```python
from build123d import *

# Parameters (mm, degrees)
SKETCH2_R           = 3
BOSS_EXTRUDE1_DEPTH = 4.7625
FILLET1_R           = 3.18


with BuildPart() as part:
    # Sketch2 → Boss-Extrude1 (new body)
    with BuildSketch(Plane.XY):
        Polygon((-31.10816412, 42.602538855), (8.89183588, 124.502538855), (48.89183588, 124.502538855), (88.89183588, 44.502538855), (88.89183588, 4.502538855), (-31.10816412, 4.502538855), align=None)
        with Locations(Location((28.89183588, 104.502538855, 0), (0, 0, 180))):
            Circle(SKETCH2_R, mode=Mode.SUBTRACT)
        with Locations(Location((28.89183588, 64.502538855, 0), (0, 0, 180))):
            Circle(SKETCH2_R, mode=Mode.SUBTRACT)
        with Locations(Location((-11.10816412, 23.552538855, 0), (0, 0, 180))):
            Circle(SKETCH2_R, mode=Mode.SUBTRACT)
        with Locations(Location((68.89183588, 23.552538855, 0), (0, 0, 180))):
            Circle(SKETCH2_R, mode=Mode.SUBTRACT)
        with Locations(Location((28.89183588, 23.552538855, 0), (0, 0, 180))):
            Circle(SKETCH2_R, mode=Mode.SUBTRACT)
    extrude(amount=BOSS_EXTRUDE1_DEPTH)

    # Fillet1
    fillet1_edges = [part.edges().sort_by_distance(p)[0] for p in [
        (-31.10816412, 42.602538855, 2.38125),
        (8.89183588, 124.502538855, 2.38125),
        (48.89183588, 124.502538855, 2.38125),
        (88.89183588, 44.502538855, 2.38125),
        (88.89183588, 4.502538855, 2.38125),
        (-31.10816412, 4.502538855, 2.38125),
    ]]
    fillet(fillet1_edges, radius=FILLET1_R)


solid = part.part
```
The model under review builds one solid part; all positions refer to its coordinate system, in mm. Give positions to 0.01 mm unless a question says otherwise; leave off trailing zeros. Order: outer loops, then holes, each group sorted by start corner. A loop starts at its lowest first (then second) coordinate and runs counter-clockwise, first axis right, second up. Notation, with made-up numbers: (24, 49) - (49, 49) arc R27 cw to (49, 83) - close; hole circle Ø10 at (20.5, 48). An arc over 180 degrees is marked (long way). Use CSV: the item, a comma, the result in double quotes. Start each with the question number.
Q1. We need section D-D, the plane y = 97.5. Write out the cut boundary in (x, z).
Q2. The part is to be moulded in two halves that separate along X. For faces 1 (the cylindrical face through (87.936, 5.409, 2.415)), 2 (the cylindrical face through (29.282, 101.528, 2.348)), 3 (the flat face through (-11.654, 82.434, 2.348)), 4 (the flat face through (30, 4.503, 2)), say which applies: +X half, -X half, draft (parallel to the pull), parting line (faces both ways), or undercut.
Q3. We need section B-B, the plane z = 1.6. Write out the cut boundary in (x, y).
Q4. To check wall thickness, follow line 1 along X through (y, z) = (67, 4.3); line 2 along X through (y, z) = (66, 3.25); line 3 along Y through (x, z) = (70.5, 2.65). State the ranges of each line that lie inside material, in increasing order. Write a range as [from, to].
Q5. We need section C-C, the plane x = 29.5. Write out the cut boundary in (y, z), and give its area (3 significant figures).
Q6. We need section A-A, the plane y = 63. Write out the cut boundary in (x, z).
Q7. Clearance check with flat-ended pins moving along their axes: pin 1 Ø3.5 at (x, y) = (28.89, 23.55) entering from +Z; pin 2 Ø1 at (y, z) = (86, 3.5) entering from +X. State where each tip first meets the part, or that it passes through.
Outcome:
1,outline,"(-4.3, 0) - (62.39, 0) - (62.39, 4.76) - (-4.3, 4.76) - close"
2,face 1,"+X half"
2,face 2,"undercut"
2,face 3,"-X half"
2,face 4,"draft"
3,outline,"(-31.11, 7.68) arc R3.18 ccw to (-27.93, 4.5) - (85.71, 4.5) arc R3.18 ccw to (88.89, 7.68) - (88.89, 43.75) arc R3.18 ccw to (88.56, 45.17) - (49.77, 122.74) arc R3.18 ccw to (46.93, 124.5) - (10.88, 124.5) arc R3.18 ccw to (8.02, 122.72) - (-30.79, 43.26) arc R3.18 ccw to (-31.11, 41.87) - close; hole circle Ø6 at (-11.11, 23.55); hole circle Ø6 at (28.89, 23.55); hole circle Ø6 at (28.89, 64.5); hole circle Ø6 at (28.89, 104.5); hole circle Ø6 at (68.89, 23.55)"
4,line 1,"x = [-19.19, 27.23], [30.55, 77.64]"
4,line 2,"x = [-19.68, 26.29], [31.49, 78.14]"
4,line 3,"y = [4.5, 21.02], [26.09, 81.29]"
5,outline,"(4.5, 0) - (20.61, 0) - (20.61, 4.76) - (4.5, 4.76) - close; (26.49, 0) - (61.56, 0) - (61.56, 4.76) - (26.49, 4.76) - close; (67.44, 0) - (101.56, 0) - (101.56, 4.76) - (67.44, 4.76) - close; (107.44, 0) - (124.5, 0) - (124.5, 4.76) - (107.44, 4.76) - close"
5,area,"488 mm^2"
6,outline,"(-21.15, 0) - (26.3, 0) - (26.3, 4.76) - (-21.15, 4.76) - close; (31.49, 0) - (79.64, 0) - (79.64, 4.76) - (31.49, 4.76) - close"
7,pin 1,"passes through"
7,pin 2,"stops at x = 68.39"
